Can you work these out from the model? Positions are in its coordinate system, mm. Face numbers are marked on the shaded views. A direction names the side the tool comes from. Give positions to 0.01 mm unless a question says otherwise; leave off trailing zeros. Order: outer loops, then holes, each group sorted by start corner. A loop starts at its lowest first (then second) coordinate and runs counter-clockwise, first axis right, second up. Notation, with made-up numbers: M -31.5,75 L 8.5,75 A29 cw 8.5,105 Z; hole C 26,53 d7. An arc over 180 degrees is marked long. Use a Markdown table: item, result. Add a question column.
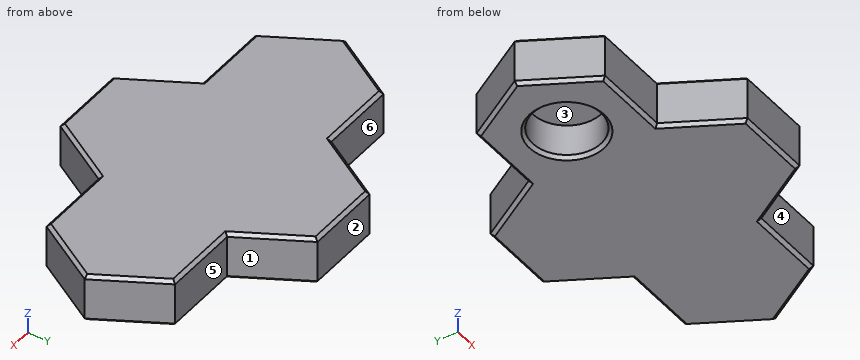
from build123d import *

# Parameters (mm, degrees)
PAD_DEPTH       = 3
SKETCH001_R     = 2.125
POCKET_DEPTH    = 2.15
CHAMFER_SIZE    = 0.2
CHAMFER001_SIZE = 0.2


with BuildPart() as part:
    # Sketch → Pad (new body)
    with BuildSketch(Plane.XY):
        Polygon((2.309401, 4), (-2.309401, 4), (-4.618802, 0), (-2.309401, -4), (2.309401, -4), (4.618802, -8), (9.237604, -8), (11.547005, -4), (16.165808, -4), (18.475209, 0), (16.165808, 4), (11.547005, 4), (9.237604, 8), (4.618802, 8), align=None)
    extrude(amount=PAD_DEPTH)

    # Sketch001 → Pocket (cut)
    with BuildSketch(Plane.XY):
        Circle(SKETCH001_R)
    extrude(amount=POCKET_DEPTH, mode=Mode.SUBTRACT)

    # Chamfer
    chamfer_edges = [part.edges().sort_by_distance(p)[0] for p in [
        (0, 4, 3),
        (-3.464102, 2, 3),
        (-3.464102, -2, 3),
        (0, -4, 3),
        (3.464102, -6, 3),
        (6.928203, -8, 3),
        (10.392305, -6, 3),
        (13.856406, -4, 3),
        (17.320508, -2, 3),
        (17.320508, 2, 3),
        (13.856406, 4, 3),
        (10.392305, 6, 3),
        (6.928203, 8, 3),
        (3.464102, 6, 3),
    ]]
    chamfer(chamfer_edges, length=CHAMFER_SIZE)

    # Chamfer001
    chamfer001_edges = [part.edges().sort_by_distance(p)[0] for p in [
        (0, 4, 0),
        (3.464102, 6, 0),
        (-3.464102, 2, 0),
        (6.928203, 8, 0),
        (-3.464102, -2, 0),
        (10.392305, 6, 0),
        (0, -4, 0),
        (13.856406, 4, 0),
        (3.464102, -6, 0),
        (17.320508, 2, 0),
        (6.928203, -8, 0),
        (17.320508, -2, 0),
        (10.392305, -6, 0),
        (13.856406, -4, 0),
        (-2.125, 0, 0),
    ]]
    chamfer(chamfer001_edges, length=CHAMFER001_SIZE)


solid = part.part
1. Will these pins go through, and if not, where does the flat tip stop? pin 1 (1.3 mm diameter, centred on x = 13.5, z = 1.5, fed in from +Y); pin 2 (0.8 mm diameter, centred on x = 1, z = 1, fed in from -Y); pin 3 (1.5 mm diameter, centred on y = -5, z = 2, fed in from -X).
2. If we section it at D-D, the plane x = 13.75: List the corners of the cut face in (y, z) for me.
3. If we section it at A-A, the plane z = 0.85: List the corners of the cut face in (x, y) for me (3 decimals), then the cut area to 3 significant figures.
4. If we section it at C-C, the plane y = -4.5: List the corners of the cut face in (x, z) for me, then the cut area to 3 significant figures.
5. If we section it at B-B, the plane x = 0: List the corners of the cut face in (y, z) for me (3 decimals), then the cut area to 3 significant figures.
6. We'd pull the mould along X, two halves only. Please class the marked faces 1, 2 and 3: +X half, -X half, draft (parallel to the pull), parting line (faces both ways), or undercut.
7. I need wall thicknesses on L1, parallel to Y at x = 0, z = 1 (3 decimals); L2, parallel to Y at x = 1.5, z = 1.9; L3, parallel to Y at x = 15.75, z = 0.8. Which ranges of each line are inside material? Lowest first, please. Write a range as [from, to].
8. On a 3-axis mill with a long thin cutter (end or side, diameter ignored), from which of +Z, -Z, +X, -X, +Y, -Y can I reach the whole of each face in a straight line? I mean the marked faces 4, 5 and 6. Say none if no direction works.
Geometry results:
| question | item | result |
|---|---|---|
| 1 | pin 1 | stops at y = 4 |
| 1 | pin 2 | stops at y = -4 |
| 1 | pin 3 | stops at x = 2.45 |
| 2 | outline | M -4,0.2 L -3.8,0 L 3.8,0 L 4,0.2 L 4,2.8 L 3.8,3 L -3.8,3 L -4,2.8 Z |
| 3 | outline | M -4.619,0 L -2.309,-4 L 2.309,-4 L 4.619,-8 L 9.238,-8 L 11.547,-4 L 16.166,-4 L 18.475,0 L 16.166,4 L 11.547,4 L 9.238,8 L 4.619,8 L 2.309,4 L -2.309,4 Z; hole C 0,0 d4.25 |
| 3 | area | 208 mm^2 |
| 4 | outline | M 2.6,0.2 L 2.83,0 L 11.03,0 L 11.26,0.2 L 11.26,2.8 L 11.03,3 L 2.83,3 L 2.6,2.8 Z |
| 4 | area | 25.9 mm^2 |
| 5 | outline | M -4,0.2 L -3.8,0 L -2.325,0 L -2.125,0.2 L -2.125,2.15 L 2.125,2.15 L 2.125,0.2 L 2.325,0 L 3.8,0 L 4,0.2 L 4,2.8 L 3.8,3 L -3.8,3 L -4,2.8 Z |
| 5 | area | 14.7 mm^2 |
| 6 | face 1 | +X half |
| 6 | face 2 | draft |
| 6 | face 3 | undercut |
| 7 | L1 | y = [-4, -2.125], [2.125, 4] |
| 7 | L2 | y = [-4, -1.51], [1.51, 4] |
| 7 | L3 | y = [-4, 4] |
| 8 | face 4 | +Z, -Z, +X, -Y |
| 8 | face 5 | +Z, -Z, +X, +Y |
| 8 | face 6 | +Z, -Z, -X, +Y |
